Source: CAD feature listing. Evaluate the final solid. Frame: model axes, mm. A direction names the side the tool comes from. Give positions to 0.01 mm unless a question says otherwise; leave off trailing zeros. Order: outer loops, then holes, each group sorted by start corner. A loop starts at its lowest first (then second) coordinate and runs counter-clockwise, first axis right, second up. Notation, with made-up numbers: (4.25, 64.5) -> (12.25, 64.5) arc R30 cw to (12.25, 99.5) -> close; hole circle Ø4 at (-30, 82). An arc over 180 degrees is marked (long way). Answer in a Markdown table with one row per item.
```python
from build123d import *

# Parameters (mm, degrees)
F0_R     = 12.7
F1_DEPTH = 2.54
F2_R     = 4.191
F3_DEPTH = 7.62
F4_R     = 2.667
F5_DEPTH = 7.621


with BuildPart() as f1:
    # F0 (on Top) → F1 (new body)
    with BuildSketch(Plane.XY):
        Circle(F0_R)
    extrude(amount=F1_DEPTH)

    # F2 (on Top) → F3 (join)
    with BuildSketch(Plane.XY):
        Circle(F2_R)
    extrude(amount=F3_DEPTH)

    # F4 (on Top) → F5 (cut, through all)
    with BuildSketch(Plane.XY):
        Circle(F4_R)
    extrude(amount=F5_DEPTH, mode=Mode.SUBTRACT)


solid = f1.part
```
(1) Ray query, probe 1 along Y at (x, z) = (0, 4.25); probe 2 along Y at (x, z) = (0, 2.5). Return the intervals inside material, ascending.
A:
| item | result |
|---|---|
| probe 1 | y = -4.19 to -2.67, 2.67 to 4.19 |
| probe 2 | y = -12.7 to -2.67, 2.67 to 12.7 |
(2) Pull-direction query (X, two-part tool) for faces 3 (the cylindrical face through (-2.75, -12.4, 1.25)), 4 (the cylindrical face through (1.231, -2.366, 3.757)), 5 (the flat face through (0, 3, 0)); classes: +X half, -X half, draft (parallel to the pull), parting line (faces both ways), or undercut.
A:
| item | result |
|---|---|
| face 3 | parting line |
| face 4 | undercut |
| face 5 | draft |
(3) Section query C-C (x = -3). Return the cut outline in (y, z), plus the area to 3 significant figures.
A:
| item | result |
|---|---|
| outline | (-12.34, 0) -> (12.34, 0) -> (12.34, 2.54) -> (2.93, 2.54) -> (2.93, 7.62) -> (-2.93, 7.62) -> (-2.93, 2.54) -> (-12.34, 2.54) -> close |
| area | 92.4 mm^2 |
(4) Section query D-D (z = 3). Return the cut outline in (x, y).
A:
| item | result |
|---|---|
| outline | circle Ø8.38 at (0, 0); hole circle Ø5.33 at (0, 0) |
(5) Access query for faces 1 (the flat face through (0, -3, 7.62)), 2 (the cylindrical face through (3.997, 1.259, 5.044)). Directions: +Z, -Z, +X, -X, +Y, -Y. A direction counts if a zero-diameter tool reaches every point of the face in a straight line with its end or side. Return the directions, or none.
A:
| item | result |
|---|---|
| face 1 | +Z, +X, -X, +Y, -Y |
| face 2 | +Z |
(6) First-contact query: pin 1 Ø4 at (x, y) = (2.5, -4) entering from -Z; pin 2 Ø4.5 at (x, y) = (0, 0) entering from -Z; pin 3 Ø1.5 at (y, z) = (-2, 1) entering from +X; pin 4 Ø1.5 at (x, z) = (-4.5, 5) entering from -Y. Flat tips, straight axial feed; report the tip coordinate or a pass-through.
A:
| item | result |
|---|---|
| pin 1 | stops at z = 0 |
| pin 2 | passes through |
| pin 3 | stops at x = 12.64 |
| pin 4 | stops at y = -1.87 |
(7) Section query A-A (y = 0). Return the cut outline in (x, z), plus the area to 3 significant figures.
A:
| item | result |
|---|---|
| outline | (-12.7, 0) -> (-2.67, 0) -> (-2.67, 7.62) -> (-4.19, 7.62) -> (-4.19, 2.54) -> (-12.7, 2.54) -> close; (2.67, 0) -> (12.7, 0) -> (12.7, 2.54) -> (4.19, 2.54) -> (4.19, 7.62) -> (2.67, 7.62) -> close |
| area | 66.5 mm^2 |
